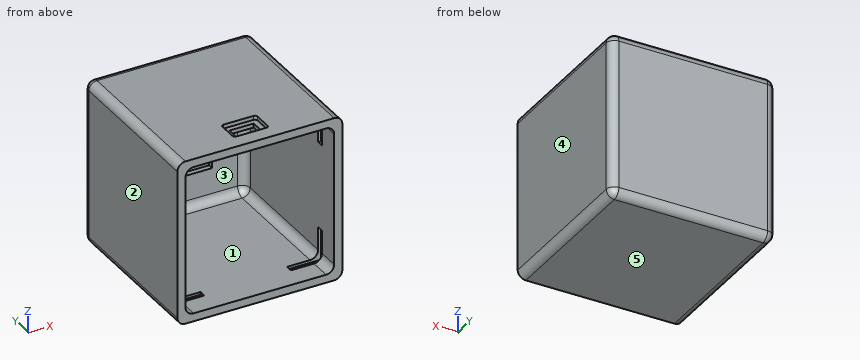
Autodesk Inventor part; units mm, degrees
ref_plane "YZ Plane" through (0, 0, 0) normal (1, 0, 0) x (0, 1, 0)
ref_plane "XZ Plane" through (0, 0, 0) normal (0, 1, 0) x (-1, 0, 0)
ref_plane "XY Plane" through (0, 0, 0) normal (0, 0, 1) x (1, 0, 0)
sketch "Эскиз1" plane through (0, 0, 0) normal (0, 1, 0) x (-1, 0, 0)
  line L0 (0, 0) -> (55, 0)
  line L1 (55, 0) -> (55, -55)
  line L2 (55, -55) -> (0, -55)
  line L3 (0, -55) -> (0, 0)
  line L4 (-3, -58) -> (58, -58)
  line L5 (58, -58) -> (58, 3)
  line L6 (58, 3) -> (-3, 3)
  line L7 (-3, 3) -> (-3, -58)
  dimension "d0" = 55
  dimension "d1" = 55
  dimension "d2" = 3
extrude "Выдавливание1" add sketch "Эскиз1" along normal blind 58
sketch "Эскиз2" plane through (0, 58, 0) normal (0, 1, 0) x (1, 0, 0)
  line L0 (-58, -3) -> (3, -3)
  line L1 (3, 58) -> (-58, 58)
  line L2 (-58, -3) -> (3, -3)
  line L3 (3, -3) -> (3, 58)
  line L4 (3, 58) -> (-58, 58)
  line L5 (-58, 58) -> (-58, -3)
  point P0 (0, 0)
  point P1 (3, -3)
extrude "Выдавливание2" add sketch "Эскиз2" along normal blind 3
sketch "Эскиз3" plane through (0, 58, 0) normal (0, -1, 0) x (1, 0, 0)
  line L0 (3, -58) -> (-58, -58)
  line L1 (-58, 3) -> (3, 3)
  line L2 (-58, -58) -> (-58, 3)
  line L3 (3, 3) -> (3, -58)
  line L4 (-42.5, -12.5) -> (-12.5, -12.5)
  line L5 (-12.5, -12.5) -> (-12.5, -42.5)
  line L6 (-12.5, -42.5) -> (-42.5, -42.5)
  line L7 (-42.5, -42.5) -> (-42.5, -12.5)
  line L8 (-42.5, -27.5) -> (-12.5, -27.5) construction
  line L9 (-27.5, -42.5) -> (-27.5, -27.5) construction
  line L10 (-55, 0) -> (-55, -55)
  line L11 (-55, -27.5) -> (0, -27.5) construction
  line L12 (0, -55) -> (0, 0)
  line L13 (-55, -55) -> (0, -55)
  line L14 (-27.5, -55) -> (-27.5, -27.5) construction
  dimension "d7" = 30
  dimension "d8" = 30
extrude "Выдавливание3" cut sketch "Эскиз3" against normal blind 2 contours L4 L5 L6 L7
ref_plane "РабПлоскость1" through (0, 8, 0) normal (0, -1, 0) x (1, 0, 0)
sketch "Эскиз4" plane through (0, 8, 0) normal (0, -1, 0) x (1, 0, 0)
  line L0 (0, -55) -> (0, 0)
  line L1 (-55, -27.5) -> (0, -27.5)
  line L2 (-27.5, -55) -> (-27.5, 0)
  line L3 (-55, 0) -> (-55, -55)
  line L4 (3, -58) -> (-58, -58)
  line L5 (3, 3) -> (3, -58)
  line L6 (-58, -58) -> (3, -58)
  line L7 (3, -58) -> (3, 3)
  line L8 (3, 3) -> (-58, 3)
  line L9 (-58, 3) -> (-58, -58)
  line L10 (-56, 1) -> (1, 1)
  line L11 (1, 1) -> (1, -56)
  line L12 (1, -56) -> (-56, -56)
  line L13 (-56, -56) -> (-56, 1)
  line L14 (-56, -56) -> (-43.5, -56)
  line L15 (-43.5, -56) -> (-43.5, -43.5)
  line L16 (-43.5, -43.5) -> (-56, -43.5)
  line L17 (-56, -43.5) -> (-56, -56)
  line L18 (-56, 1) -> (-43.5, 1)
  line L19 (-43.5, 1) -> (-43.5, -11.5)
  line L20 (-43.5, -11.5) -> (-56, -11.5)
  line L21 (-56, -11.5) -> (-56, 1)
  line L22 (1, -56) -> (-11.5, -56)
  line L23 (-11.5, -56) -> (-11.5, -43.5)
  line L24 (-11.5, -43.5) -> (1, -43.5)
  line L25 (1, -43.5) -> (1, -56)
  line L26 (-11.5, 1) -> (-11.5, -11.5)
  line L27 (1, 1) -> (-11.5, 1)
  line L28 (-11.5, -11.5) -> (1, -11.5)
  line L29 (1, -11.5) -> (1, 1)
  point P0 (-11.5, 1)
  point P1 (1, -11.5)
  point P2 (1, -43.5)
  point P3 (-11.5, -56)
  point P4 (-56, -11.5)
  point P5 (-43.5, 1)
  point P6 (-56, -43.5)
  point P7 (-43.5, -56)
  dimension "d14" = 2
  dimension "d15" = 12.5
  dimension "d16" = 12.5
extrude "Выдавливание4" cut sketch "Эскиз4" against normal blind 2.5 contours L24 L11 L12 L23 | L28 L26 L10 L11 | L12 L13 L16 L15 | L20 L13 L10 L19
fillet "Сопряжение1" radius 3 16 edges at (-55, 34.25, 0) (0, 34.25, 0) (0, 34.25, -55) (-55, 34.25, -55) (3, 30.5, 3) (-58, 30.5, 3) (-58, 30.5, -58) (-58, 61, -27.5) (-27.5, 61, -58) (3, 61, -27.5) (3, 30.5, -58) (-27.5, 61, 3) (-27.5, 58, -55) (-55, 58, -27.5) (-27.5, 58, 0) (0, 58, -27.5)
fillet "Сопряжение2" radius 3 4 edges at (0, 4, -55) (-55, 4, -55) (-55, 4, 0) (0, 4, 0)
sketch "Эскиз5" plane through (-55, 0, 3) normal (0, 0, 1) x (1, 0, 0)
  line L0 (55, 8) -> (55, 10.5)
  line L1 (0, 8) -> (0, 10.5)
  line L2 (55, 8) -> (0, 8)
  line L3 (27.5, 8) -> (27.5, 13.4815) construction
  line L4 (27.5, 8) -> (27.5, 7.5) construction
  line L5 (23, 12) -> (32, 12)
  line L6 (32, 12) -> (32, 7.5)
  line L7 (32, 7.5) -> (23, 7.5)
  line L8 (23, 7.5) -> (23, 12)
  point P0 (55, 0)
  point P1 (27.5, 12)
  dimension "d27" = 0.5
  dimension "d28" = 9
  dimension "d29" = 4.5
extrude "Выдавливание5" cut sketch "Эскиз5" against normal blind 3
sketch "Эскиз8" plane through (-55, 0, 3) normal (0, 0, 1) x (1, 0, 0)
  line L0 (32, 12) -> (32, 7.5)
  line L1 (23, 12) -> (32, 12)
  line L2 (32, 7.5) -> (23, 7.5)
  line L3 (23, 7.5) -> (23, 12)
  line L4 (23, 12) -> (32, 12)
  line L5 (32, 12) -> (32, 7.5)
  line L6 (22, 5.5) -> (33, 5.5)
  line L7 (34, 6.5) -> (34, 13)
  line L8 (33, 14) -> (22, 14)
  line L9 (21, 13) -> (21, 6.5)
  arc A0 (33, 5.5) -> (34, 6.5) centre (33, 6.5) ccw
  arc A1 (34, 13) -> (33, 14) centre (33, 13) ccw
  arc A2 (22, 14) -> (21, 13) centre (22, 13) ccw
  arc A3 (21, 6.5) -> (22, 5.5) centre (22, 6.5) ccw
  point P0 (55, 0)
  dimension "d40" = 2
  dimension "d41" = 1
extrude "Выдавливание6" cut sketch "Эскиз8" against normal blind 1.5
sketch "Эскиз9" plane through (0, 0, -58) normal (0, 0, -1) x (-1, 0, 0)
  line L0 (3.8898, 30.331) -> (51.1102, 30.331) construction
  line L1 (51.1102, 30.331) -> (51.1102, 16.9712) construction
  line L2 (51.1102, 16.9712) -> (3.8898, 16.9712) construction
  line L3 (3.8898, 16.9712) -> (3.8898, 30.331) construction
  line L4 (12.5, 58) -> (42.5, 58)
  line L5 (27.5, 58) -> (27.5, 0) construction
  line L6 (0, 0) -> (55, 0)
  point P0 (27.5, 30.331)
equation "\"d8\" = d7"
equation "\"d16\" = d15"
properties part number "box"
Can you work these out from the model? Positions are in its coordinate system, mm. Face numbers are marked on the shaded views. A direction names the side the tool comes from. Round coordinates to 2 decimals unless told otherwise and drop trailing zeros. Write each loop counter-clockwise with the first axis right and the second up, starting at its lowest first coordinate (ties: lowest second). Pieces come first, ordered by that corner, then holes. Notation, with made-up numbers: (50.5, 57.25) -> (91.5, 57.25) arc R18 cw to (91.5, 73.25) -> close; hole circle Ø7 at (-7.75, 39.5). An arc over 180 degrees is marked (long way). Use one line per item in the form item = value. Start each with the question number.
Q1. Imagine slicing it at C-C (z = -17). Please give me the cut outline in (x, y).
Q2. If I drill on probe 1 along X at (y, z) = (42, -29); probe 2 along X at (y, z) = (46, -54), over which ranges is the centre line in solid material (lowest first)? Write a range as [from, to].
Q3. We'd pull the mould along X, two halves only. Please class the marked faces 3, 4 and 5: +X half, -X half, draft (parallel to the pull), parting line (faces both ways), or undercut.
Q4. Imagine slicing it at A-A (x = -26). Please give me the cut outline in (y, z).
Q5. I'm going to push flat-ended pins straight in: P1, Ø0.5, axis at x = -55.5, y = 8.5, coming from the -Z side; P2, Ø2, axis at x = -32.5, z = -19, coming from the -Y side; P3, Ø4, axis at x = -47.5, z = -47.5, coming from the -Y side. Where does each tip first touch, or does it pass through?
Q6. Imagine slicing it at D-D (x = -8.5). Please give me the cut outline in (y, z), then the cut area to 3 significant figures.
Q7. Imagine slicing it at B-B (y = 16). Please give me the cut outline in (x, z).
Q8. Which directions (+Z, -Z, +X, -X, +Y, -Y) give clear straight access to the entire face, cutting with the end or side of a thin tool? Please do the marked faces 1 and 2.
Worked out:
q1.outline = (-58, 0) -> (-55, 0) -> (-55, 55) arc R3 cw to (-52, 58) -> (-42.5, 58) -> (-42.5, 60) -> (-12.5, 60) -> (-12.5, 58) -> (-3, 58) arc R3 cw to (0, 55) -> (0, 0) -> (3, 0) -> (3, 58) arc R3 ccw to (0, 61) -> (-55, 61) arc R3 ccw to (-58, 58) -> close
q2.probe_1 = [-58, -55], [0, 3]
q2.probe_2 = [-58, -54.24], [-0.76, 3]
q3.face_3 = undercut
q3.face_4 = +X half
q3.face_5 = draft
q4.outline = (0, -58) -> (58, -58) arc R3 ccw to (61, -55) -> (61, 0) arc R3 ccw to (58, 3) -> (14, 3) -> (14, 1.5) -> (12, 1.5) -> (12, 0) -> (55, 0) arc R3 cw to (58, -3) -> (58, -12.5) -> (60, -12.5) -> (60, -42.5) -> (58, -42.5) -> (58, -52) arc R3 cw to (55, -55) -> (0, -55) -> close; (0, 0) -> (7.5, 0) -> (7.5, 1.5) -> (5.5, 1.5) -> (5.5, 3) -> (0, 3) -> close
q5.P1 = -57.99
q5.P2 = 60
q5.P3 = 58
q6.outline = (0, -58) -> (58, -58) arc R3 ccw to (61, -55) -> (61, 0) arc R3 ccw to (58, 3) -> (0, 3) -> (0, 0) -> (8, 0) -> (8, 1) -> (10.5, 1) -> (10.5, 0) -> (55, 0) arc R3 cw to (58, -3) -> (58, -52) arc R3 cw to (55, -55) -> (10.5, -55) -> (10.5, -56) -> (8, -56) -> (8, -55) -> (0, -55) -> close
q6.area = 526 mm^2
q7.outline = (-58, -55) arc R3 ccw to (-55, -58) -> (0, -58) arc R3 ccw to (3, -55) -> (3, 0) arc R3 ccw to (0, 3) -> (-55, 3) arc R3 ccw to (-58, 0) -> close; hole (-55, -52) arc R3 ccw to (-52, -55) -> (-3, -55) arc R3 ccw to (0, -52) -> (0, -3) arc R3 ccw to (-3, 0) -> (-52, 0) arc R3 ccw to (-55, -3) -> close
q8.face_1 = -Y
q8.face_2 = +Z, -Z, -X, +Y, -Y
